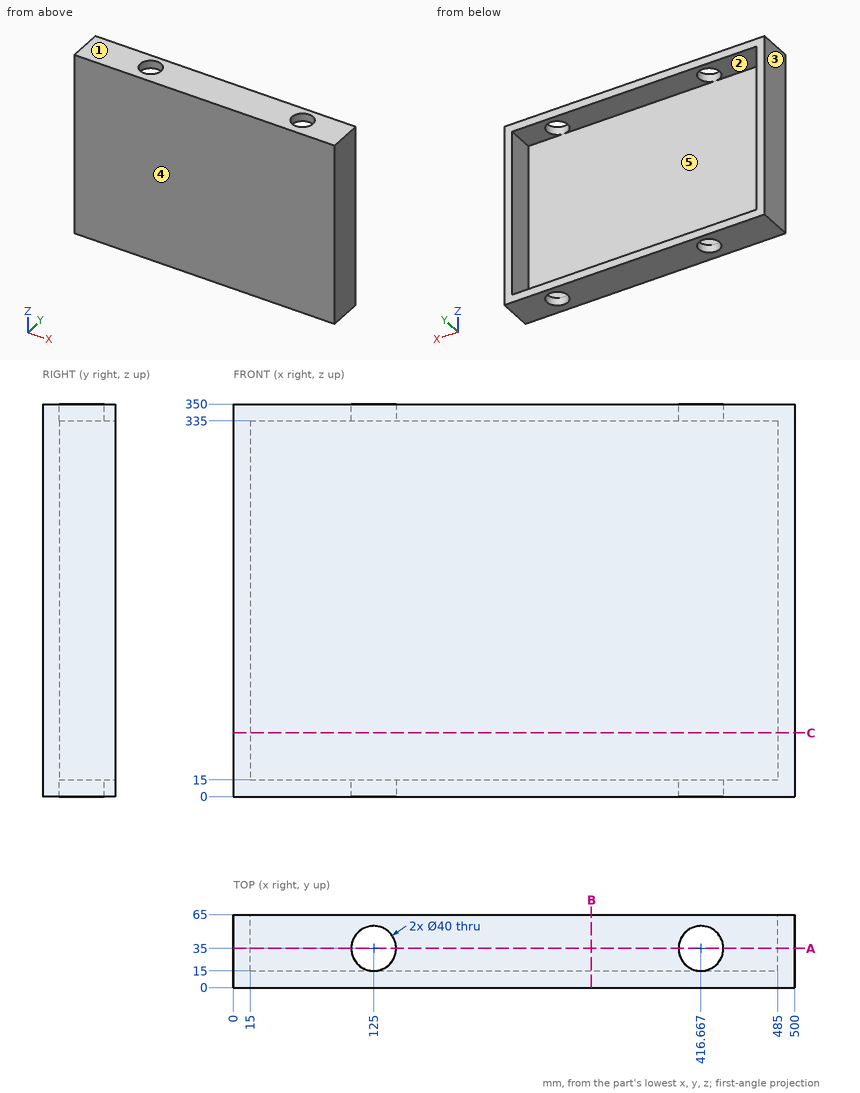
Print and shaded views of the part. All mm, measured from the part's lowest x, y and z. A direction names the side the tool comes from. Coordinates: 2 decimals unless noted, no trailing zeros. Order: outer loops, then holes, each group sorted by start corner. A loop starts at its lowest first (then second) coordinate and runs counter-clockwise, first axis right, second up. Notation, with made-up numbers: M 60.25,30.25 L 110.25,30.25 A11 ccw 110.25,39.25 Z; hole C 20,81.25 d4. An arc over 180 degrees is marked long. One line per question, with ' | ' between items. Start each with the question number.
Q1. 3-axis set-ups, long thin cutter, end or side, ignore diameter. For the marked faces 1 and 2: which of +Z, -Z, +X, -X, +Y, -Y reach the whole face in a straight line?
Q2. Saw through at B-B (x = 319). List the corners of the cut face in (y, z).
Q3. Probe L1, parallel to X at y = 35, z = 343.75; L2, parallel to X at y = 50, z = 306; L3, parallel to Z at x = 99.5, y = 32. List the from-to ranges inside material, lowest first. Write a range as from..to.
Q4. Saw through at A-A (y = 35). List the corners of the cut face in (x, z), then the cut area to 3 significant figures.
Q5. Two-plate mould, pull along X, no slides. Class the marked faces 3, 4 and 5: +X half, -X half, draft (parallel to the pull), parting line (faces both ways), or undercut.
Q6. Saw through at C-C (z = 57). List the corners of the cut face in (x, y).
Q7. Flat gauge pins, fed straight in: pin 1 Ø10 at (x, z) = (140.5, 270) entering from -Y; pin 2 Ø24 at (x, y) = (416.67, 35) entering from +Z; pin 3 Ø1 at (x, z) = (60, 145) entering from +Y. Where does each tip first touch, or does it go through?
Check values:
1) face 1: +Z, +X, -X, +Y, -Y | face 2: +Y
2) outline: M 0,0 L 65,0 L 65,15 L 15,15 L 15,335 L 65,335 L 65,350 L 0,350 Z
3) L1: x = 0..105, 145..396.67, 436.67..500 | L2: x = 0..15, 485..500 | L3: z = 0..15, 335..350
4) outline: M 0,0 L 105,0 L 105,15 L 15,15 L 15,335 L 105,335 L 105,350 L 0,350 Z; M 145,0 L 396.67,0 L 396.67,15 L 145,15 Z; M 145,335 L 396.67,335 L 396.67,350 L 145,350 Z; M 436.67,0 L 500,0 L 500,350 L 436.67,350 L 436.67,335 L 485,335 L 485,15 L 436.67,15 Z | area: 22,200 mm2
5) face 3: -X half | face 4: draft | face 5: undercut
6) outline: M 0,0 L 500,0 L 500,65 L 485,65 L 485,15 L 15,15 L 15,65 L 0,65 Z
7) pin 1: stops at y = 0 | pin 2: passes through | pin 3: stops at y = 15
